For this review, take the finished solid that the model builds, in its own axes (mm). A direction names the side the tool comes from. Round coordinates to 2 decimals unless told otherwise and drop trailing zeros. Loops run counter-clockwise (first coordinate to the right, second up) from the corner with the lowest first, then second, coordinate; pieces in that order, holes last. Notation, with made-up numbers: (0, 63) -> (35, 63) arc R30 ccw to (35, 96) -> close; hole circle Ø10 at (-18.5, 13.25). An arc over 180 degrees is marked (long way). Write each question's results on one line, items separated by ' | '.
```python
from build123d import *

# Parameters (mm, degrees)
SKETCH1_W           = 177.8
SKETCH1_H           = 38.1
SKETCH1_W_2         = 38.1
SKETCH1_H_2         = 88.9
BOSS_EXTRUDE1_DEPTH = 25.4
SKETCH2_R           = 9.525
CUT_EXTRUDE1_DEPTH  = 26.4
SKETCH3_R           = 9.525
CUT_EXTRUDE2_DEPTH  = 26.4


with BuildPart() as part:
    # Sketch1 → Boss-Extrude1 (new body)
    with BuildSketch(Plane.XY):
        with Locations((88.9, 19.05)):
            Rectangle(SKETCH1_W, SKETCH1_H)
        with Locations((158.75, -44.45)):
            Rectangle(SKETCH1_W_2, SKETCH1_H_2)
    extrude(amount=BOSS_EXTRUDE1_DEPTH)

    # Sketch2 → Cut-Extrude1 (cut, through all)
    with BuildSketch(Plane.XY.offset(25.4)):
        with Locations((25.4, 19.05)):
            Circle(SKETCH2_R)
    extrude(amount=-CUT_EXTRUDE1_DEPTH, mode=Mode.SUBTRACT)

    # Sketch3 → Cut-Extrude2 (cut, through all)
    with BuildSketch(Plane.XY.offset(25.4)):
        with Locations((158.75, -63.5)):
            Circle(SKETCH3_R)
    extrude(amount=-CUT_EXTRUDE2_DEPTH, mode=Mode.SUBTRACT)


solid = part.part
```
1. To check wall thickness, follow probe 1 along Y at (x, z) = (158.75, 7.25) (3 decimals); probe 2 along Y at (x, z) = (25.4, 15) (3 decimals); probe 3 along Y at (x, z) = (61, 5.25). State the ranges of each line that lie inside material, in increasing order.
Values found:
probe 1: y = -88.9 to -73.025, -53.975 to 38.1 | probe 2: y = 0 to 9.525, 28.575 to 38.1 | probe 3: y = 0 to 38.1
2. Consider section A-A (y = -63.5). State the section outline as (x, z) points (3 decimals), plus the area to 3 significant figures.
Values found:
outline: (139.7, 0) -> (149.225, 0) -> (149.225, 25.4) -> (139.7, 25.4) -> close; (168.275, 0) -> (177.8, 0) -> (177.8, 25.4) -> (168.275, 25.4) -> close | area: 484 mm2
3. Consider section C-C (z = 19.5). State the section outline as (x, y) points (3 decimals), plus the area to 3 significant figures.
Values found:
outline: (0, 0) -> (139.7, 0) -> (139.7, -88.9) -> (177.8, -88.9) -> (177.8, 38.1) -> (0, 38.1) -> close; hole circle Ø19.05 at (25.4, 19.05); hole circle Ø19.05 at (158.75, -63.5) | area: 9,590 mm2
4. Consider section B-B (x = 158.75). State the section outline as (y, z) points (3 decimals).
Values found:
outline: (-88.9, 0) -> (-73.025, 0) -> (-73.025, 25.4) -> (-88.9, 25.4) -> close; (-53.975, 0) -> (38.1, 0) -> (38.1, 25.4) -> (-53.975, 25.4) -> close
5. For pin 1 (1.5 mm diameter, centred on x = 84, z = 22.5, fed in from -Y); pin 2 (2 mm diameter, centred on y = -42, z = 22.5, fed in from -X), all flat-tipped, find the tip position at first contact; note any pin that passes through.
Values found:
pin 1: stops at y = 0 | pin 2: stops at x = 139.7
6. Tool access review of faces 1 (the face through (158, -88.9, 13)), 2 (the face through (139.7, -45, 13)): name each direction out of +Z, -Z, +X, -X, +Y, -Y from which nothing blocks a thin tool from reaching the whole face with its end or side.
Values found:
face 1: +Z, -Z, +X, -X, -Y | face 2: +Z, -Z, -X, -Y
7. Consider section D-D (x = 125.5). State the section outline as (y, z) points, plus the area to 3 significant figures.
Values found:
outline: (0, 0) -> (38.1, 0) -> (38.1, 25.4) -> (0, 25.4) -> close | area: 968 mm2
8. Draft analysis for pull direction X (two halves, no side actions). For faces 3 (the face through (69, 0, 13)), 4 (the face through (0, 19, 13)), 5 (the face through (177.8, -26, 13)), 6 (the face through (149.234, -63.081, 12.878)), state which applies: released by +X, released by -X, zero draft, split by the parting line, or undercut.
Values found:
face 3: zero draft | face 4: released by -X | face 5: released by +X | face 6: undercut
